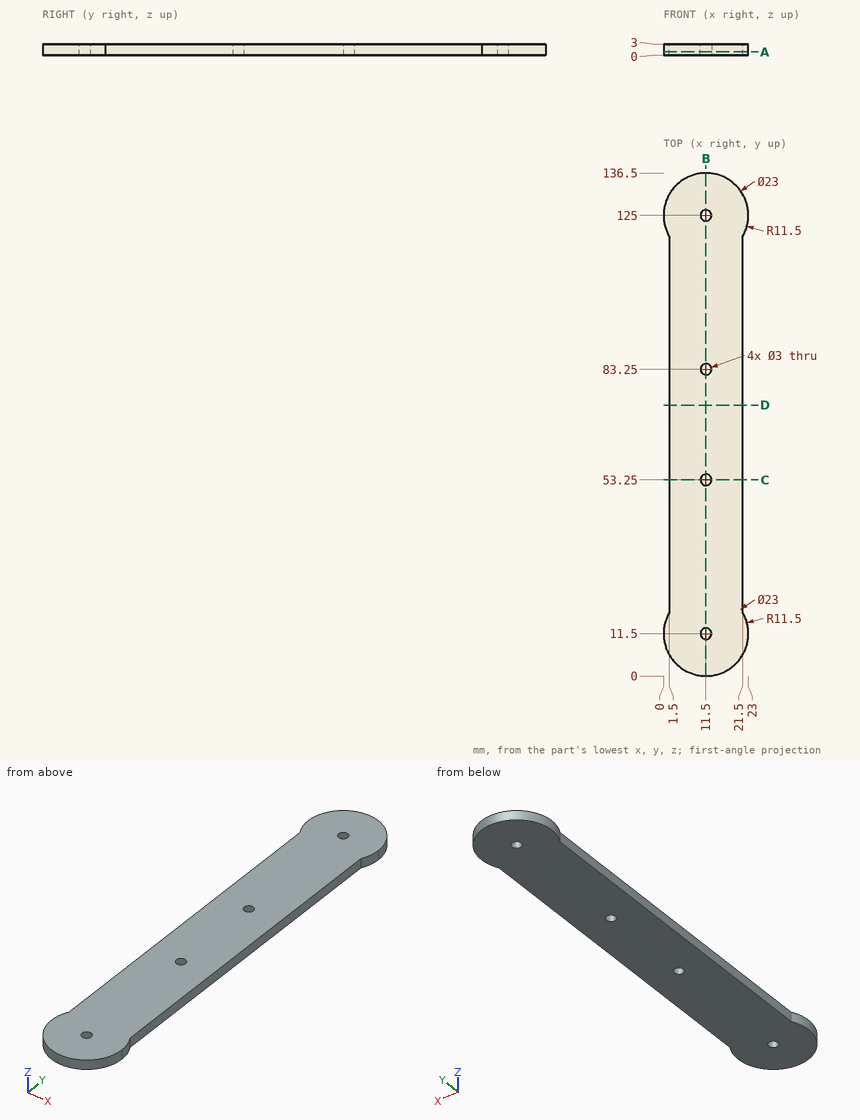
The figure shows three views and two pictorial views of one solid part (mm, origin at its lowest corner). Answer the questions. Coordinates: 2 decimals unless noted, no trailing zeros. Write each loop counter-clockwise with the first axis right and the second up, starting at its lowest first coordinate (ties: lowest second). Pieces come first, ordered by that corner, then holes.
1. The part is cut by section D-D, the plane y = 73.5. Write down the section's boundary in (x, z), and give its area (3 significant figures).
Results list:
outline: (1.5, 0) - (21.5, 0) - (21.5, 3) - (1.5, 3) - close
area: 60.0 mm2
2. The part is cut by section A-A, the plane z = 0.85. Write down the section's boundary in (x, y), and give its area (3 significant figures).
Results list:
outline: (1.5, 17.18) arc R11.5 ccw (long way) to (21.5, 17.18) - (21.5, 119.32) arc R11.5 ccw (long way) to (1.5, 119.32) - close; hole circle Ø3 at (11.5, 11.5); hole circle Ø3 at (11.5, 53.25); hole circle Ø3 at (11.5, 83.25); hole circle Ø3 at (11.5, 125)
area: 2,680 mm2
3. Flat-ended cylindrical pins translate along their axes: pin 1 (1.5 mm diameter, centred on x = 15.5, z = 1.5, fed in from -Y); pin 2 (1.5 mm diameter, centred on x = 12.5, z = 1.5, fed in from +Y). Find the tip coordinate at first contact, or state that the pin passes through.
Results list:
pin 1: stops at y = 0.47
pin 2: stops at y = 136.5
4. The part is cut by section C-C, the plane y = 53.25. Write down the section's boundary in (x, z), and give its area (3 significant figures).
Results list:
outline: (1.5, 0) - (10, 0) - (10, 3) - (1.5, 3) - close; (13, 0) - (21.5, 0) - (21.5, 3) - (13, 3) - close
area: 51.0 mm2
5. Consider line 1 along Y through (x, z) = (11.5, 0.8); line 2 along X through (y, z) = (53, 2.05); line 3 along X through (y, z) = (125, 1.9). Determine where each line is inside the solid, lowest interval first.
Results list:
line 1: y = 0 to 10, 13 to 51.75, 54.75 to 81.75, 84.75 to 123.5, 126.5 to 136.5
line 2: x = 1.5 to 10.02, 12.98 to 21.5
line 3: x = 0 to 10, 13 to 23
6. The part is cut by section B-B, the plane x = 11.5. Write down the section's boundary in (y, z), and give its area (4 significant figures).
Results list:
outline: (0, 0) - (10, 0) - (10, 3) - (0, 3) - close; (13, 0) - (51.75, 0) - (51.75, 3) - (13, 3) - close; (54.75, 0) - (81.75, 0) - (81.75, 3) - (54.75, 3) - close; (84.75, 0) - (123.5, 0) - (123.5, 3) - (84.75, 3) - close; (126.5, 0) - (136.5, 0) - (136.5, 3) - (126.5, 3) - close
area: 373.5 mm2
